Geometry check sheet. Reference: the model listing, model coordinates, mm. A direction names the side the tool comes from. Round coordinates to 2 decimals unless told otherwise and drop trailing zeros. Order: outer loops, then holes, each group sorted by start corner. A loop starts at its lowest first (then second) coordinate and runs counter-clockwise, first axis right, second up. Notation, with made-up numbers: (-10, -24.75) - (22, -24.75) arc R15 cw to (22, -16.75) - close; hole circle Ø9 at (82.25, 21). An arc over 180 degrees is marked (long way). Return JSON: item names as keys, results as strings. Group by question number.
Q1. Sectioned sample at D-D, the plane x = 87.5. Record the cut outline in (y, z), then the cut area to 3 significant figures.
Q2. Sectioned sample at C-C, the plane z = 1.5. Give the number of separate pieces and of enclosed holes in the cut face, then the cut area to 3 significant figures.
Q3. Sectioned sample at B-B, the plane x = 40. Record the cut outline in (y, z), then the cut area to 3 significant figures.
Q4. Sectioned sample at A-A, the plane x = 17. Record the cut outline in (y, z).
Q5. Gauge pin test, flat ends, axial feed: pin 1 Ø1.8 at (x, y) = (87.5, 0) entering from +Z; pin 2 Ø5 at (x, y) = (40, -3.5) entering from +Z; pin 3 Ø1 at (y, z) = (3.5, 1.5) entering from +X; pin 4 Ø10.5 at (x, y) = (80, 0) entering from +Z. Record the tip position at first contact, or that the pin passes through.
Q6. Draft check along Y on faces 3 (the cylindrical face through (38.5, -3.57, 1.48)), 4 (the flat face through (41, 10, 1)), 5 (the flat face through (39, 0, 0)). Enter one of: pulls with the +Y half, pulls with the -Y half, needs draft (parallel to the pull), parting line crosses it, or undercut.
Q7. Material ranges on line 1 along X through (y, z) = (-4.25, 2.65); line 2 along Y through (x, z) = (0, 0.4); line 3 along Y through (x, z) = (63, 1.95), recorded low to high.
Q8. Tool access check on faces 1 (the cylindrical face through (64.43, -0.45, 1.48)), 2 (the cylindrical face through (74.505, 0.242, 2.014)). Record the directions out of +Z, -Z, +X, -X, +Y, -Y that give a thin tool (end or side, any length) a straight path to the whole face; none if there is none.
Autodesk Inventor part; units mm, degrees
ref_plane "YZ Plane" through (0, 0, 0) normal (1, 0, 0) x (0, 1, 0)
ref_plane "XZ Plane" through (0, 0, 0) normal (0, 1, 0) x (-1, 0, 0)
ref_plane "XY Plane" through (0, 0, 0) normal (0, 0, 1) x (1, 0, 0)
sketch "Sketch1" plane through (0, 0, 0) normal (0, 0, 1) x (1, 0, 0)
  line L0 (0, 0) -> (80, 0) construction
  line L1 (0, -10) -> (80, -10)
  line L2 (80, 10) -> (0, 10)
  arc A0 (0, 10) -> (0, -10) centre (0, 0) ccw
  arc A1 (80, -10) -> (80, 10) centre (80, 0) ccw
  line L3 (0, 0) -> (80, 0) construction
  circle A2 centre (0, 0) radius 4
  circle A3 centre (80, 0) radius 4
  circle A4 centre (40, 3.5) radius 1.5
  circle A5 centre (40, -3.5) radius 1.5
  circle A6 centre (87.5, 0) radius 1.5
  circle A7 centre (-7.5, 0) radius 1.5
  circle A8 centre (17, 0) radius 1.5
  circle A9 centre (63, 0) radius 1.5
  point P0 (40, 0)
  point P1 (40, 0)
  dimension "d0" = 80
  dimension "d1" = 0
  dimension "d2" = 20
  dimension "d3" = 8
  dimension "d4" = 8
  dimension "d5" = 3
  dimension "d6" = 3
  dimension "d7" = 3
  dimension "d8" = 3
  dimension "d9" = 0
  dimension "d10" = 7.5
  dimension "d11" = 0
  dimension "d12" = 7.5
  dimension "d13" = 3
  dimension "d14" = 3
  dimension "d15" = 3.5
  dimension "d16" = 3.5
  dimension "d17" = 17
  dimension "d18" = 17
  dimension "d19" = 0
  dimension "d20" = 0
extrude "Extrusion1" add sketch "Sketch1" along normal blind 3
sketch "Sketch2" plane through (0, 0, 3) normal (0, 0, 1) x (1, 0, 0)
  circle A0 centre (0, 0) radius 4
  circle A1 centre (80, 0) radius 4
  circle A2 centre (0, 0) radius 5.5
  circle A3 centre (80, 0) radius 5.5
  dimension "d23" = 11
  dimension "d24" = 11
extrude "Extrusion2" cut sketch "Sketch2" against normal blind 2 contours A0 | A1 | A2 | A3
properties part number "Arm4" material "Aluminum 6061, Welded"
Reply:
{
 "1": {"outline": "(-6.61, 0) - (-1.5, 0) - (-1.5, 3) - (-6.61, 3) - close; (1.5, 0) - (6.61, 0) - (6.61, 3) - (1.5, 3) - close", "area": "30.7 mm^2"},
 "2": {"separate pieces": "1", "enclosed holes": "8", "area": "1,680 mm^2"},
 "3": {"outline": "(-10, 0) - (-5, 0) - (-5, 3) - (-10, 3) - close; (-2, 0) - (2, 0) - (2, 3) - (-2, 3) - close; (5, 0) - (10, 0) - (10, 3) - (5, 3) - close", "area": "42.0 mm^2"},
 "4": {"outline": "(-10, 0) - (-1.5, 0) - (-1.5, 3) - (-10, 3) - close; (1.5, 0) - (10, 0) - (10, 3) - (1.5, 3) - close"},
 "5": {"pin 1": "through", "pin 2": "z = 3", "pin 3": "x = 89.54", "pin 4": "z = 1"},
 "6": {"face 3": "undercut", "face 4": "pulls with the +Y half", "face 5": "needs draft"},
 "7": {"line 1": "-9.05 to -3.49, 3.49 to 38.7, 41.3 to 76.51, 83.49 to 89.05", "line 2": "-10 to -4, 4 to 10", "line 3": "-10 to -1.5, 1.5 to 10"},
 "8": {"face 1": "+Z, -Z", "face 2": "+Z"}
}
